from build123d import *

# Parameters (mm, degrees)
SKETCH_1_W          = 127.5
SKETCH_1_H          = 185
SKETCH_1_R          = 1.6
EXTRUDE_1_DEPTH     = 1
SKETCH_2_W          = 127.5
SKETCH_2_H          = 35
EXTRUDE_2_DEPTH     = 1
SKETCH_3_R          = 1.6
CUT_EXTRUDE_1_DEPTH = 10
SKETCH_4_W          = 127.5
SKETCH_4_H          = 3
CUT_EXTRUDE_2_DEPTH = 10
SKETCH_5_W          = 22
SKETCH_5_H          = 17
CUT_EXTRUDE_3_DEPTH = 10
FILLET_2_R          = 2


with BuildPart() as part:
    # 草图1 → 凸台-拉伸1 (new body)
    with BuildSketch(Plane.XY):
        Rectangle(SKETCH_1_W, SKETCH_1_H)
        with Locations((-21.5, 89.5)):
            Circle(SKETCH_1_R, mode=Mode.SUBTRACT)
        with Locations((-1.5, 89.5)):
            Circle(SKETCH_1_R, mode=Mode.SUBTRACT)
        with Locations((-60.75, 15)):
            Circle(SKETCH_1_R, mode=Mode.SUBTRACT)
        with Locations((-60.75, -5)):
            Circle(SKETCH_1_R, mode=Mode.SUBTRACT)
    extrude(amount=EXTRUDE_1_DEPTH)

    # 草图2 → 凸台-拉伸2 (add)
    with BuildSketch(Plane.XY.offset(1)):
        with Locations((0, -110)):
            Rectangle(SKETCH_2_W, SKETCH_2_H)
    extrude(amount=-EXTRUDE_2_DEPTH)

    # 草图3 → 切除-拉伸1 (cut)
    with BuildSketch(Plane(origin=(0, 0, 0), x_dir=(-1, 0, 0), z_dir=(0, 0, -1))):
        with Locations((-7, -117.4)):
            Circle(SKETCH_3_R)
        with Locations((7, -117.4)):
            Circle(SKETCH_3_R)
    extrude(amount=-CUT_EXTRUDE_1_DEPTH, mode=Mode.SUBTRACT)

    # 草图4 → 切除-拉伸2 (cut)
    with BuildSketch(Plane(origin=(0, 0, 0), x_dir=(-1, 0, 0), z_dir=(0, 0, -1))):
        with Locations((0, -126)):
            Rectangle(SKETCH_4_W, SKETCH_4_H)
    extrude(amount=-CUT_EXTRUDE_2_DEPTH, mode=Mode.SUBTRACT)

    # 草图5 → 切除-拉伸3 (cut)
    with BuildSketch(Plane.XY.offset(1)):
        with Locations((52.75, -116)):
            Rectangle(SKETCH_5_W, SKETCH_5_H)
    extrude(amount=-CUT_EXTRUDE_3_DEPTH, mode=Mode.SUBTRACT)

    # 圆角2
    fillet_2_edges = [part.edges().sort_by_distance(p)[0] for p in [
        (-63.75, -124.5, 0.5),
        (41.75, -124.5, 0.5),
        (-63.75, 92.5, 0.5),
        (63.75, 92.5, 0.5),
        (63.75, -107.5, 0.5),
        (41.75, -107.5, 0.5),
    ]]
    fillet(fillet_2_edges, radius=FILLET_2_R)


solid = part.part
Geometry check sheet. Reference: the model listing, model coordinates, mm. Give positions to 0.01 mm unless a question says otherwise; leave off trailing zeros. Loops run counter-clockwise (first coordinate to the right, second up) from the corner with the lowest first, then second, coordinate; pieces in that order, holes last. Notation, with made-up numbers: M -39,79.25 L -29,79.25 A4 ccw -29,85.25 Z; hole C 59.25,-38.75 d10. An arc over 180 degrees is marked long. Write each question's results on one line, items separated by ' | '.
1) Thickness scan on line 1 (X direction, y = 89.5, z = 0.2); line 2 (X direction, y = -117.4, z = 0.35); line 3 (Y direction, x = -21.5, z = 0.45). Record the ranges inside material, lowest first.
Answers follow:
line 1: -63.75 to -23.1, -19.9 to -3.1, 0.1 to 63.75 | line 2: -63.75 to -8.6, -5.4 to 5.4, 8.6 to 41.75 | line 3: -124.5 to 87.9, 91.1 to 92.5
2) Gauge pin test, flat ends, axial feed: pin 1 (0.5 mm diameter, centred on x = 54.5, z = 0.5, fed in from -Y); pin 2 (3 mm diameter, centred on x = -1.5, y = 89.5, fed in from +Z). Record the tip position at first contact, or that the pin passes through.
Answers follow:
pin 1: y = -107.5 | pin 2: through
3) Section check A-A, the plane z = 0.55. Record the boundary of the cut face in (x, y).
Answers follow:
outline: M -63.75,-122.5 A2 ccw -61.75,-124.5 L 39.75,-124.5 A2 ccw 41.75,-122.5 L 41.75,-109.5 A2 cw 43.75,-107.5 L 61.75,-107.5 A2 ccw 63.75,-105.5 L 63.75,90.5 A2 ccw 61.75,92.5 L -61.75,92.5 A2 ccw -63.75,90.5 Z; hole C -60.75,-5 d3.2; hole C -60.75,15 d3.2; hole C -21.5,89.5 d3.2; hole C -7,-117.4 d3.2; hole C -1.5,89.5 d3.2; hole C 7,-117.4 d3.2
4) Section check B-B, the plane x = 47.5. Record the boundary of the cut face in (y, z).
Answers follow:
outline: M -107.5,0 L 92.5,0 L 92.5,1 L -107.5,1 Z
